```python
from build123d import *

# Parameters (mm, degrees)
F0_R      = 25.4
F1_DEPTH  = 25.4
F2_W      = 25.4
F2_H      = 50.8
F3_DEPTH  = 101.6
F4_W      = 19.05
F4_H      = 44.45
F5_DEPTH  = 101.6
F6_R      = 22.225
F7_DEPTH  = 22.225
F9_DEPTH  = 3.175
F11_DEPTH = 3.175
F13_DEPTH = 50.8


with BuildPart() as f1:
    # F0 (on Front) → F1 (new body)
    with BuildSketch(Plane.XZ):
        Circle(F0_R)
    extrude(amount=-F1_DEPTH)

    # F2 (on Right) → F3 (join)
    with BuildSketch(Plane.YZ):
        with Locations((12.7, 0)):
            Rectangle(F2_W, F2_H)
    extrude(amount=-F3_DEPTH)

    # F4 (on face) → F5 (cut)
    with BuildSketch(Plane(origin=(-101.6, 0, 0), x_dir=(0, -1, 0), z_dir=(-1, 0, 0))):
        with Locations((-12.7, 0)):
            Rectangle(F4_W, F4_H)
    extrude(amount=-F5_DEPTH, mode=Mode.SUBTRACT)

    # F6 (on face) → F7 (cut)
    with BuildSketch(Plane(origin=(0, 25.4, 0), x_dir=(-1, 0, 0), z_dir=(0, 1, 0))):
        Circle(F6_R)
    extrude(amount=-F7_DEPTH, mode=Mode.SUBTRACT)

    # F8 (on face) → F9 (join)
    with BuildSketch(Plane(origin=(0, 0, -25.4), x_dir=(1, 0, 0), z_dir=(0, 0, -1))):
        Polygon((-127, 0), (-101.6, -25.4), (-101.6, 0), align=None)
    extrude(amount=-F9_DEPTH)

    # F10 (on face) → F11 (join)
    with BuildSketch(Plane.XY.offset(25.4)):
        Polygon((-101.6, 0), (-101.6, 25.4), (-127, 0), align=None)
    extrude(amount=-F11_DEPTH)

    # F12 (on face) → F13 (join)
    with BuildSketch(Plane.XY.offset(25.4)):
        Polygon((-97.109872, 25.4), (-101.6, 25.4), (-127, 0), (-122.509872, 0), align=None)
    extrude(amount=-F13_DEPTH)


solid = f1.part
```
Geometry check sheet. Reference: the model listing, model coordinates, mm. A direction names the side the tool comes from. Round coordinates to 2 decimals unless told otherwise and drop trailing zeros. Loops run counter-clockwise (first coordinate to the right, second up) from the corner with the lowest first, then second, coordinate; pieces in that order, holes last. Notation, with made-up numbers: (75.5, 66.25) -> (107.5, 66.25) arc R24 ccw to (107.5, 92.25) -> close; hole circle Ø9 at (66.5, 72.25). An arc over 180 degrees is marked (long way). Use a Markdown table: item, result.
(1) Sectioned sample at D-D (x = -20.5). Enter the section's corners in (y, z) (3 decimals).
Calculated:
| item | result |
|---|---|
| outline | (0, -25.4) -> (25.4, -25.4) -> (25.4, -8.585) -> (22.225, -8.585) -> (22.225, -22.225) -> (3.175, -22.225) -> (3.175, 22.225) -> (22.225, 22.225) -> (22.225, 8.585) -> (25.4, 8.585) -> (25.4, 25.4) -> (0, 25.4) -> close |
(2) Sectioned sample at B-B (x = -59.5). Enter the section's corners in (y, z) (3 decimals), then the cut area to 3 significant figures.
Calculated:
| item | result |
|---|---|
| outline | (0, -25.4) -> (25.4, -25.4) -> (25.4, 25.4) -> (0, 25.4) -> close; hole (3.175, -22.225) -> (22.225, -22.225) -> (22.225, 22.225) -> (3.175, 22.225) -> close |
| area | 444 mm² |
(3) Set-up check for faces 1 (the flat face through (-101.6, 2, 0)), 2 (the flat face through (-35, 0, 0)), 3 (the flat face through (-64, 13, 25.4)), 4 (the cylindrical face through (22.204, 14.443, 0.977)), 5 (the flat face through (-62, 22.225, 0)): record each of +Z, -Z, +X, -X, +Y, -Y from which the full face is reachable in a straight line by a thin tool's end or side.
Calculated:
| item | result |
|---|---|
| face 1 | -Y |
| face 2 | +Z, -Z, +X, -X, -Y |
| face 3 | +Z, +X, -X, +Y, -Y |
| face 4 | +Y |
| face 5 | none |
(4) Go/stop test with flat-tipped pins: P1, Ø1.6, axis at y = 1, z = -8.5, coming from the -X side; P2, Ø3, axis at y = 7, z = -1, coming from the -X side; P3, Ø3, axis at x = -106.5, z = -17.5, coming from the -Y side. Record where each tip stops, or that it passes through.
Calculated:
| item | result |
|---|---|
| P1 | x = -126.8 |
| P2 | x = -121.5 |
| P3 | y = 14.51 |
(5) Sectioned sample at A-A (z = 0). Enter the section's corners in (x, y) (3 decimals), then the cut area to 3 significant figures.
Calculated:
| item | result |
|---|---|
| outline | (-127, 0) -> (-122.51, 0) -> (-100.285, 22.225) -> (-22.225, 22.225) -> (-22.225, 25.4) -> (-101.6, 25.4) -> close; (-101.6, 0) -> (25.4, 0) -> (25.4, 25.4) -> (22.225, 25.4) -> (22.225, 3.175) -> (-101.6, 3.175) -> close |
| area | 831 mm² |
(6) Sectioned sample at C-C (y = 20). Enter the section's corners in (x, z) (3 decimals), then the cut area to 3 significant figures.
Calculated:
| item | result |
|---|---|
| outline | (-107, -25.4) -> (0, -25.4) arc R25.4 ccw to (0, 25.4) -> (-107, 25.4) -> close; hole (-102.51, -22.225) -> (0, -22.225) arc R22.225 ccw to (0, 22.225) -> (-102.51, 22.225) -> close |
| area | 1,120 mm² |
(7) Scan lines: probe 1 along Y at (x, z) = (-85.5, 15.5) (3 decimals); probe 2 along Z at (x, y) = (-62.5, 13.75) (3 decimals); probe 3 along Y at (x, z) = (12.5, 16) (3 decimals). Record each from-to range of solid material in increasing order.
Calculated:
| item | result |
|---|---|
| probe 1 | 0 to 3.175, 22.225 to 25.4 |
| probe 2 | -25.4 to -22.225, 22.225 to 25.4 |
| probe 3 | 0 to 3.175 |
(8) Mould release check, pull along Y, two halves, no side actions. Record for faces 6 (the flat face through (-114, 13, 0)), 7 (the flat face through (-64, 13, -25.4)), 8 (the flat face through (-41, 3.175, 0)): released by +Y, released by -Y, zero draft, split by the parting line, or undercut.
Calculated:
| item | result |
|---|---|
| face 6 | released by +Y |
| face 7 | zero draft |
| face 8 | undercut |
